Source: CAD feature listing. Evaluate the final solid. Frame: model axes, mm. Coordinates: 2 decimals unless noted, no trailing zeros. Order: outer loops, then holes, each group sorted by start corner. A loop starts at its lowest first (then second) coordinate and runs counter-clockwise, first axis right, second up.
```python
from build123d import *

# Parameters (mm, degrees)
SKETCH1_R           = 139.7
SKETCH1_R_2         = 84.1375
BOSS_EXTRUDE1_DEPTH = 12.7
SKETCH2_W           = 11.176
SKETCH2_H           = 12.7
CIRPATTERN1_COUNT   = 8


with BuildPart() as part:
    # Sketch1 → Boss-Extrude1 (new body)
    with BuildSketch(Plane.XY):
        Circle(SKETCH1_R)
        Circle(SKETCH1_R_2, mode=Mode.SUBTRACT)
    extrude(amount=BOSS_EXTRUDE1_DEPTH)

    # Sketch2 → 7/8 (0.88) Diameter Hole1 (revolve, cut)
    with BuildSketch(Plane(origin=(120.65, 0, 12.7), x_dir=(0, -1, 0), z_dir=(1, 0, 0))):
        with Locations((5.588, 6.35)):
            Rectangle(SKETCH2_W, SKETCH2_H)
    f_7_8_0_88_diameter_hole1 = revolve(axis=Axis((120.65, 0, 19.05), (0, 0, -1)), mode=Mode.SUBTRACT)

    # CirPattern1: 7/8 (0.88) Diameter Hole1 ×8 about axis
    cirpattern1_axis = Axis((0, 0, 0), (0, 0, 1))
    for i in range(1, CIRPATTERN1_COUNT):
        add(f_7_8_0_88_diameter_hole1.rotate(cirpattern1_axis, i * 360 / CIRPATTERN1_COUNT), mode=Mode.SUBTRACT)


solid = part.part
```
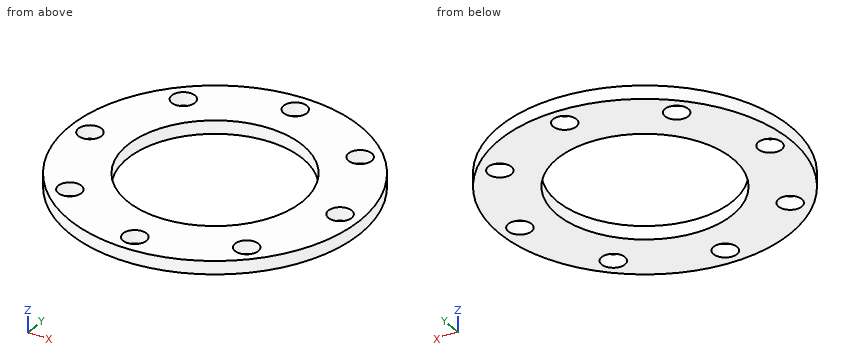
Q1. Section query A-A on y = 0. Output: boundary loops of the cut face in (x, z), plus the area to 3 significant figures.
Solutions:
outline: (-139.7, 0) - (-131.83, 0) - (-131.83, 12.7) - (-139.7, 12.7) - close; (-109.47, 0) - (-84.14, 0) - (-84.14, 12.7) - (-109.47, 12.7) - close; (84.14, 0) - (109.47, 0) - (109.47, 12.7) - (84.14, 12.7) - close; (131.83, 0) - (139.7, 0) - (139.7, 12.7) - (131.83, 12.7) - close
area: 844 mm2
Q2. Material intervals for line 1 along Y through (x, z) = (0, 10.25); line 2 along X through (y, z) = (0.5, 1.25); line 3 along Y through (x, z) = (-122, 3.5), sorted ascending.
Solutions:
line 1: y = -139.7 to -131.83, -109.47 to -84.14, 84.14 to 109.47, 131.83 to 139.7
line 2: x = -139.7 to -131.81, -109.49 to -84.14, 84.14 to 109.49, 131.81 to 139.7
line 3: y = -68.06 to -11.09, 11.09 to 68.06
Q3. Section query C-C on x = -113. Output: boundary loops of the cut face in (y, z), plus the area to 3 significant figures.
Solutions:
outline: (-82.14, 0) - (-8.15, 0) - (-8.15, 12.7) - (-82.14, 12.7) - close; (8.15, 0) - (82.14, 0) - (82.14, 12.7) - (8.15, 12.7) - close
area: 1,880 mm2
Q4. Pin query (flat end, axial travel): P1, Ø5, axis at x = -7.5, z = 3.5, coming from the -Y side; P2, Ø4, axis at x = -83.5, z = 3, coming from the +Y side; P3, Ø5, axis at x = -59.5, z = 8.5, coming from the -Y side. Return the tip coordinate at first contact, or that it passes through.
Solutions:
P1: stops at y = -139.61
P2: stops at y = 113.46
P3: stops at y = -127.54
Q5. Section query D-D on z = 8.25. Give the number of separate pieces and of enclosed holes in the cut face, plus the area to 3 significant figures.
Solutions:
separate pieces: 1
enclosed holes: 9
area: 35,900 mm2
